Verification items for this drawing (mm, ordinates from the low corner). A direction names the side the tool comes from. Round coordinates to 2 decimals unless told otherwise and drop trailing zeros. Loops run counter-clockwise (first coordinate to the right, second up) from the corner with the lowest first, then second, coordinate; pieces in that order, holes last. Notation, with made-up numbers: M 17.5,-34 L 65.5,-34 A16 ccw 65.5,-18 Z; hole C -22.75,-37 d10. An arc over 180 degrees is marked long. Answer as CSV lines item,"result".
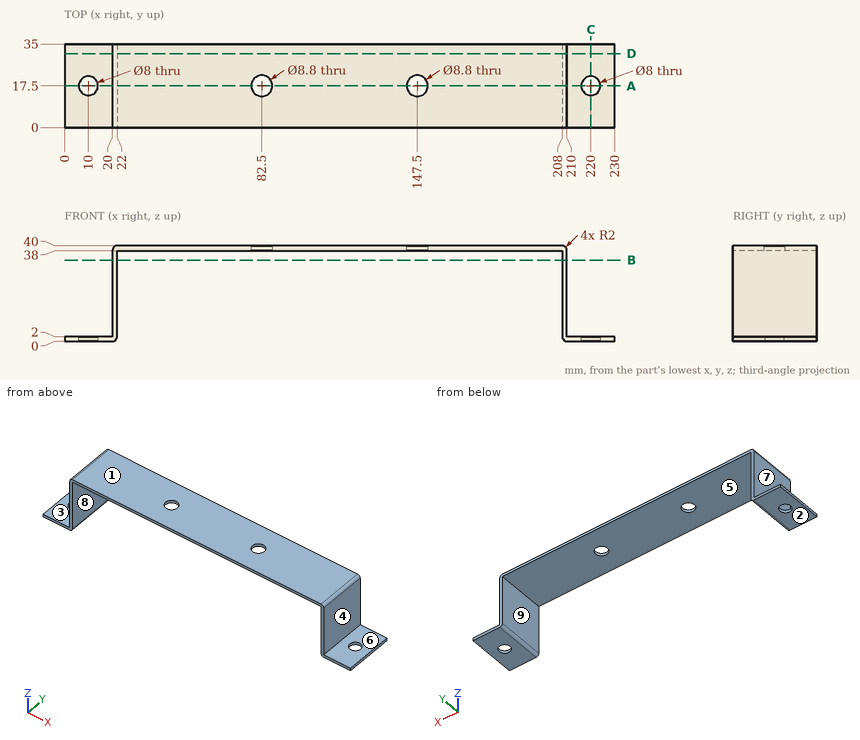
1) Section check A-A (y = 17.5). State how many separate pieces and enclosed holes the cut face has, plus the area to 3 significant figures.
Here are the results:
separate pieces,"5"
enclosed holes,"0"
area,"541 mm^2"
2) Section check B-B (z = 34). Record the cut outline in (x, y).
Here are the results:
outline,"M 20,0 L 22,0 L 22,35 L 20,35 Z; M 208,0 L 210,0 L 210,35 L 208,35 Z"
3) Section check D-D (y = 31). Record the cut outline in (x, z).
Here are the results:
outline,"M 0,0 L 20,0 A2 ccw 22,2 L 22,38 L 208,38 L 208,2 A2 ccw 210,0 L 230,0 L 230,2 L 210,2 L 210,38 A2 ccw 208,40 L 22,40 A2 ccw 20,38 L 20,2 L 0,2 Z"
4) Draft check along X on the marked faces 6, 7, 8 and 9. Enter one of: +X half, -X half, draft (parallel to the pull), parting line (faces both ways), or undercut.
Here are the results:
face 6,"draft"
face 7,"-X half"
face 8,"undercut"
face 9,"undercut"
5) Material ranges on probe 1 along Y at (x, z) = (82.5, 39); probe 2 along X at (y, z) = (6, 15); probe 3 along Y at (x, z) = (10, 0.95), recorded low to high.
Here are the results:
probe 1,"y = 0 to 13.1, 21.9 to 35"
probe 2,"x = 20 to 22, 208 to 210"
probe 3,"y = 0 to 13.5, 21.5 to 35"
6) Set-up check for the marked faces 1, 2, 3, 4 and 5: record each of +Z, -Z, +X, -X, +Y, -Y from which the full face is reachable in a straight line by a thin tool's end or side.
Here are the results:
face 1,"+Z, +X, -X, +Y, -Y"
face 2,"-Z, +X, -X, +Y, -Y"
face 3,"+Z, -X, +Y, -Y"
face 4,"+Z, +X, +Y, -Y"
face 5,"-Z, +Y, -Y"
7) Go/stop test with flat-tipped pins: pin 1 (5.5 mm diameter, centred on x = 147.5, y = 17.5, fed in from +Z); pin 2 (8 mm diameter, centred on x = 172.5, y = 5.5, fed in from -Z); pin 3 (8 mm diameter, centred on y = 17.5, z = 7.5, fed in from -X); pin 4 (17.5 mm diameter, centred on y = 13.5, z = 21.5, fed in from +X). Record where each tip stops, or that it passes through.
Here are the results:
pin 1,"passes through"
pin 2,"stops at z = 38"
pin 3,"stops at x = 20"
pin 4,"stops at x = 210"
8) Section check C-C (x = 220). Record the cut outline in (y, z).
Here are the results:
outline,"M 0,0 L 13.5,0 L 13.5,2 L 0,2 Z; M 21.5,0 L 35,0 L 35,2 L 21.5,2 Z"
